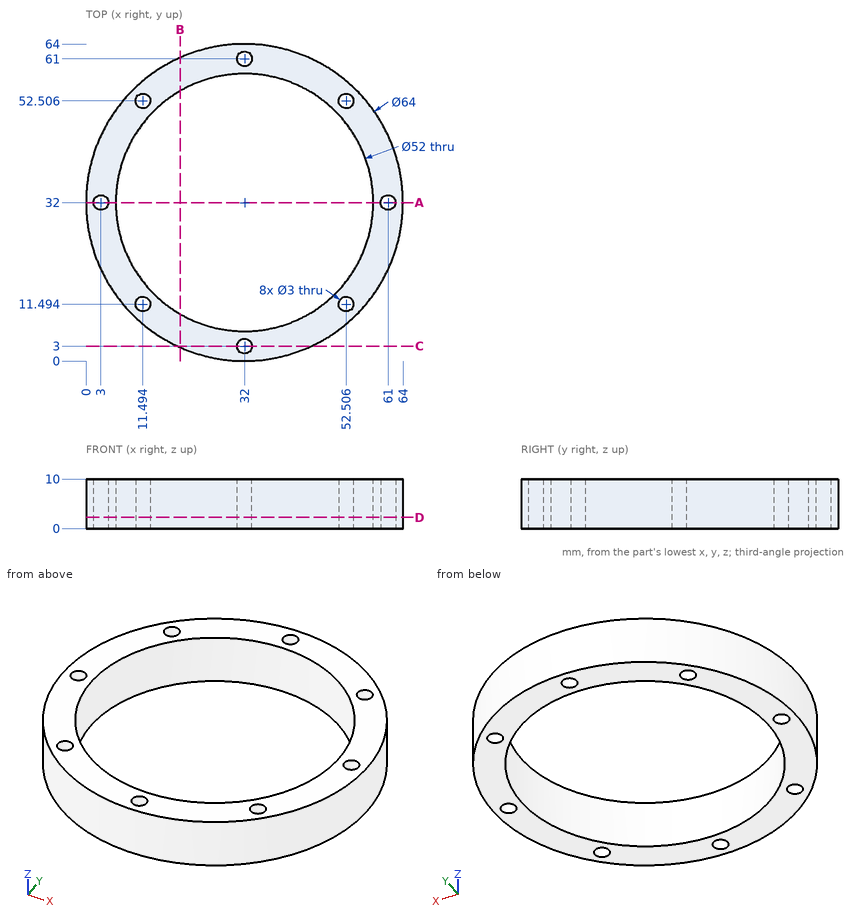
The figure shows three views and two pictorial views of one solid part (mm, origin at its lowest corner). Answer the questions. Give positions to 0.01 mm unless a question says otherwise; leave off trailing zeros. Write each loop counter-clockwise with the first axis right and the second up, starting at its lowest first coordinate (ties: lowest second). Pieces come first, ordered by that corner, then holes.
Q1. The part is cut by section C-C on y = 3. Give the vertices of the cut face in (x, z).
Answer:
outline: (18.47, 0) - (30.5, 0) - (30.5, 10) - (18.47, 10) - close; (33.5, 0) - (45.53, 0) - (45.53, 10) - (33.5, 10) - close
Q2. The part is cut by section D-D on z = 2.25. State how many separate pieces and enclosed holes the cut face has, and give its area (3 significant figures).
Answer:
separate pieces: 1
enclosed holes: 9
area: 1,040 mm2
Q3. Given pin 1 (4 mm diameter, centred on x = 12.5, z = 2, fed in from -Y); pin 2 (4 mm diameter, centred on y = 45.5, z = 9, fed in from +X); pin 3 (1 mm diameter, centred on x = 54, z = 5.5, fed in from -Y), each flat-ended and moving along its own axis, determine where each tip first touches the part or whether it passes through.
Answer:
pin 1: stops at y = 5.21
pin 2: stops at x = 61.86
pin 3: stops at y = 8.3
Q4. Straight lines are drawn through the part: L1, parallel to Y at x = 32, z = 5; L2, parallel to Y at x = 38, z = 0.75; L3, parallel to Y at x = 48.5, z = 9.25. For each, find the intervals that lie inside material, in ascending order.
Answer:
L1: y = 0 to 1.5, 4.5 to 6, 58 to 59.5, 62.5 to 64
L2: y = 0.57 to 6.7, 57.3 to 63.43
L3: y = 4.58 to 11.91, 52.09 to 59.42
Q5. The part is cut by section B-B on x = 19. Give the vertices of the cut face in (y, z), and give its area (3 significant figures).
Answer:
outline: (2.76, 0) - (9.48, 0) - (9.48, 10) - (2.76, 10) - close; (54.52, 0) - (61.24, 0) - (61.24, 10) - (54.52, 10) - close
area: 134 mm2
Q6. The part is cut by section A-A on y = 32. Give the vertices of the cut face in (x, z).
Answer:
outline: (0, 0) - (1.5, 0) - (1.5, 10) - (0, 10) - close; (4.5, 0) - (6, 0) - (6, 10) - (4.5, 10) - close; (58, 0) - (59.5, 0) - (59.5, 10) - (58, 10) - close; (62.5, 0) - (64, 0) - (64, 10) - (62.5, 10) - close
